Read the model definition and answer for the solid it produces. Units are mm, in the model's axes. Give positions to 0.01 mm unless a question says otherwise; leave off trailing zeros. Order: outer loops, then holes, each group sorted by start corner. A loop starts at its lowest first (then second) coordinate and runs counter-clockwise, first axis right, second up. Notation, with made-up numbers: (63, -18.5) - (96, -18.5) arc R25 ccw to (96, 4.5) - close; hole circle Ø11 at (64.5, 50). An arc over 180 degrees is marked (long way). One line per item, written item: value. Start each with the question number.
```python
from build123d import *

# Parameters (mm, degrees)
SKETCH_1_R          = 135
SKETCH_1_R_2        = 2
SKETCH_1_W          = 40
SKETCH_1_H          = 62
SKETCH_1_R_3        = 1.75
EXTRUDE_1_DEPTH     = 3
FILLET_1_R          = 5
SKETCH_2_R          = 20
SKETCH_2_R_2        = 2
SKETCH_2_R_3        = 1.6
SKETCH_2_W          = 30
SKETCH_2_H          = 8
SKETCH_2_W_2        = 10
SKETCH_2_H_2        = 38.624758258
CUT_EXTRUDE_1_DEPTH = 10
FILLET_2_R          = 4


with BuildPart() as part:
    # 草图1 → 凸台-拉伸1 (new body)
    with BuildSketch(Plane.XY):
        Circle(SKETCH_1_R)
        with Locations((-14.4, -110.804246301)):
            Circle(SKETCH_1_R_2, mode=Mode.SUBTRACT)
        with Locations((-20, -99.304246301)):
            Circle(SKETCH_1_R_2, mode=Mode.SUBTRACT)
        with Locations((-14.4, -87.804246301)):
            Circle(SKETCH_1_R_2, mode=Mode.SUBTRACT)
        with Locations((14.4, -110.804246301)):
            Circle(SKETCH_1_R_2, mode=Mode.SUBTRACT)
        with Locations((14.4, -87.804246301)):
            Circle(SKETCH_1_R_2, mode=Mode.SUBTRACT)
        with Locations((20, -99.304246301)):
            Circle(SKETCH_1_R_2, mode=Mode.SUBTRACT)
        with Locations((-86, 49.65212315)):
            Rectangle(SKETCH_1_W, SKETCH_1_H, mode=Mode.SUBTRACT)
        with Locations((-53, 34.65212315)):
            Circle(SKETCH_1_R_3, mode=Mode.SUBTRACT)
        with Locations((-53, 64.65212315)):
            Circle(SKETCH_1_R_3, mode=Mode.SUBTRACT)
        with Locations((-29, 34.65212315)):
            Circle(SKETCH_1_R_3, mode=Mode.SUBTRACT)
        with Locations((-29, 64.65212315)):
            Circle(SKETCH_1_R_3, mode=Mode.SUBTRACT)
        with Locations((29, 34.65212315)):
            Circle(SKETCH_1_R_3, mode=Mode.SUBTRACT)
        with Locations((29, 64.65212315)):
            Circle(SKETCH_1_R_3, mode=Mode.SUBTRACT)
        with Locations((53, 34.65212315)):
            Circle(SKETCH_1_R_3, mode=Mode.SUBTRACT)
        with Locations((53, 64.65212315)):
            Circle(SKETCH_1_R_3, mode=Mode.SUBTRACT)
        with Locations((86, 49.65212315)):
            Rectangle(SKETCH_1_W, SKETCH_1_H, mode=Mode.SUBTRACT)
    extrude(amount=EXTRUDE_1_DEPTH)

    # 圆角1
    fillet_1_edges = [part.edges().sort_by_distance(p)[0] for p in [
        (66, 80.65212315, 1.5),
        (66, 18.65212315, 1.5),
        (106, 18.65212315, 1.5),
        (106, 80.65212315, 1.5),
        (-106, 80.65212315, 1.5),
        (-106, 18.65212315, 1.5),
        (-66, 18.65212315, 1.5),
        (-66, 80.65212315, 1.5),
    ]]
    fillet(fillet_1_edges, radius=FILLET_1_R)

    # 草图2 → 切除-拉伸1 (cut)
    with BuildSketch(Plane.XY.offset(3)):
        Circle(SKETCH_2_R)
        with Locations((-72, 97)):
            Circle(SKETCH_2_R_2)
        with Locations((72, 97)):
            Circle(SKETCH_2_R_2)
        with Locations((72, -97)):
            Circle(SKETCH_2_R_2)
        with Locations((-72, -97)):
            Circle(SKETCH_2_R_2)
        with Locations((-60, 94)):
            Circle(SKETCH_2_R_3)
        with Locations((-60, 14)):
            Circle(SKETCH_2_R_3)
        with Locations((-40, 94)):
            Circle(SKETCH_2_R_3)
        with Locations((-40, 14)):
            Circle(SKETCH_2_R_3)
        with Locations((60, 14)):
            Circle(SKETCH_2_R_3)
        with Locations((60, 94)):
            Circle(SKETCH_2_R_3)
        with Locations((40, 94)):
            Circle(SKETCH_2_R_3)
        with Locations((40, 14)):
            Circle(SKETCH_2_R_3)
        with Locations((38.142857143, -10)):
            Rectangle(SKETCH_2_W, SKETCH_2_H)
        with Locations((-38.142857143, -10)):
            Rectangle(SKETCH_2_W, SKETCH_2_H)
        with Locations((38.142857143, -80)):
            Rectangle(SKETCH_2_W, SKETCH_2_H)
        with Locations((-38.142857143, -80)):
            Rectangle(SKETCH_2_W, SKETCH_2_H)
        with Locations((60, -45)):
            Rectangle(SKETCH_2_W_2, SKETCH_2_H_2)
        with Locations((-60, -45)):
            Rectangle(SKETCH_2_W_2, SKETCH_2_H_2)
        with BuildLine():
            Line((-36.755588957, 121.9), (36.755588957, 121.9))
            ThreePointArc((36.755588957, 121.9), (38.655588957, 120), (36.755588957, 118.1))
            Line((36.755588957, 118.1), (-36.755588957, 118.1))
            ThreePointArc((-36.755588957, 118.1), (-38.655588957, 120), (-36.755588957, 121.9))
        make_face()
        with BuildLine():
            Line((-36.755588957, -118.1), (36.755588957, -118.1))
            ThreePointArc((36.755588957, -118.1), (38.655588957, -120), (36.755588957, -121.9))
            Line((36.755588957, -121.9), (-36.755588957, -121.9))
            ThreePointArc((-36.755588957, -121.9), (-38.655588957, -120), (-36.755588957, -118.1))
        make_face()
        with BuildLine():
            Line((20, 101), (-20, 101))
            ThreePointArc((-20, 101), (-24, 97), (-20, 93))
            Line((-20, 93), (20, 93))
            ThreePointArc((20, 93), (24, 97), (20, 101))
        make_face()
    extrude(amount=-CUT_EXTRUDE_1_DEPTH, mode=Mode.SUBTRACT)

    # 圆角2
    fillet_2_edges = [part.edges().sort_by_distance(p)[0] for p in [
        (-53.142857143, -84, 1.5),
        (-23.142857143, -84, 1.5),
        (-53.142857143, -76, 1.5),
        (-23.142857143, -76, 1.5),
        (23.142857143, -84, 1.5),
        (23.142857143, -76, 1.5),
        (53.142857143, -76, 1.5),
        (53.142857143, -84, 1.5),
        (-53.142857143, -14, 1.5),
        (-53.142857143, -6, 1.5),
        (-23.142857143, -14, 1.5),
        (-23.142857143, -6, 1.5),
        (23.142857143, -14, 1.5),
        (53.142857143, -14, 1.5),
        (23.142857143, -6, 1.5),
        (53.142857143, -6, 1.5),
        (-55, -64.312379129, 1.5),
        (-65, -64.312379129, 1.5),
        (55, -64.312379129, 1.5),
        (65, -64.312379129, 1.5),
        (-65, -25.687620871, 1.5),
        (-55, -25.687620871, 1.5),
        (65, -25.687620871, 1.5),
        (55, -25.687620871, 1.5),
    ]]
    fillet(fillet_2_edges, radius=FILLET_2_R - 0.0001)  # a hair under: the kernel refuses the full size


solid = part.part
```
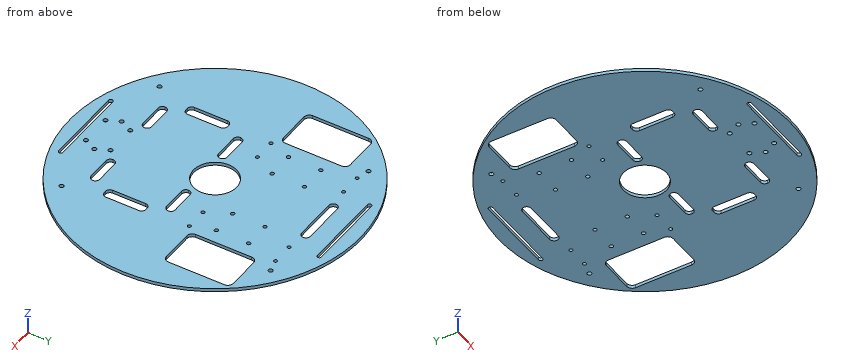
1) Section B-B on x = 89.5 is taken. Write down the section's boundary in (y, z), plus the area to 3 significant figures.
2) Each of these flat-tipped pins is pushed along its axis until it touches: pin 1 (0.6 mm diameter, centred on x = -59.5, z = 1, fed in from +Y); pin 2 (2.5 mm diameter, centred on x = -60, y = 94, fed in from +Z); pin 3 (1.5 mm diameter, centred on y = -47, z = 1, fed in from -X); pin 4 (1.5 mm diameter, centred on y = -79.5, z = 2, fed in from -X). Where does it stop, or does it pass through?
3) Section C-C on y = 58 is taken. Write down the section's boundary in (x, z).
4) Section A-A on y = 0 is taken. Write down the section's boundary in (x, z), plus the area to 3 significant figures.
5) Section D-D on z = 2.3 is taken. Give the number of separate pieces and of enclosed holes in the cut face, plus the area to 3 significant figures.
6) Find the intervals of material crossed by probe 1 along X at (y, z) = (-32.5, 2.25); probe 2 along Y at (x, z) = (31, 0.3); probe 3 along X at (y, z) = (20.5, 2.55), in increasing order. Write a range as from..to.
Solved:
1. outline: (-101.07, 0) - (18.65, 0) - (18.65, 3) - (-101.07, 3) - close; (80.65, 0) - (101.07, 0) - (101.07, 3) - (80.65, 3) - close
1. area: 420 mm2
2. pin 1: stops at y = 121.33
2. pin 2: passes through
2. pin 3: stops at x = -126.83
2. pin 4: stops at x = -109.65
3. outline: (-121.91, 0) - (-106, 0) - (-106, 3) - (-121.91, 3) - close; (-66, 0) - (66, 0) - (66, 3) - (-66, 3) - close; (106, 0) - (121.91, 0) - (121.91, 3) - (106, 3) - close
4. outline: (-135, 0) - (-20, 0) - (-20, 3) - (-135, 3) - close; (20, 0) - (135, 0) - (135, 3) - (20, 3) - close
4. area: 690 mm2
5. separate pieces: 1
5. enclosed holes: 38
5. area: 48,200 mm2
6. probe 1: x = -131.03..-65, -55..55, 65..131.03
6. probe 2: y = -131.39..-121.9, -118.1..-84, -76..-14, -6..118.1, 121.9..131.39
6. probe 3: x = -133.43..-104.88, -67.12..67.12, 104.88..133.43
